The model under review builds one solid part; all positions refer to its coordinate system, in mm. A direction names the side the tool comes from. Coordinates: 2 decimals unless noted, no trailing zeros. Write each loop counter-clockwise with the first axis right and the second up, starting at its lowest first coordinate (ties: lowest second). Pieces come first, ordered by that corner, then holes. Notation, with made-up numbers: (55, 86) - (85, 86) arc R21 cw to (85, 94) - close; hole circle Ø2 at (79.5, 58.25). An arc over 180 degrees is marked (long way). Return JSON: item names as keys, results as strings. Group by question number.
(1) To check wall thickness, follow L1, parallel to Y at x = 0, z = 6.35; L2, parallel to X at y = 55, z = 25.5; L3, parallel to Z at x = 2, y = 54. State the ranges of each line that lie inside material, in increasing order. Write a range as from..to.
(2) We need section D-D on x = 13. State the section outline as (y, z) points, then the cut area to 3 significant figures.
(3) Tool access review of faces 5 (the face through (-29, 33.924, 4)), 6 (the face through (0, 43, 4.25)), 7 (the face through (10.25, 34, 31)): name each direction out of +Z, -Z, +X, -X, +Y, -Y from which nothing blocks a thin tool from reaching the whole face with its end or side.
(4) Draft analysis for pull direction Y (two halves, no side actions). For faces 1 (the face through (-27.766, 32.006, 32.728)), 2 (the face through (-10.25, 34, 4)), 3 (the face through (1.344, 38.032, 29.197)), 4 (the face through (29, 33.924, 4)), state which applies: released by +Y, released by -Y, zero draft, split by the parting line, or undercut.
(5) We need section B-B on z = 17.5. Give the number of separate pieces and of enclosed holes in the cut face, then the cut area to 3 significant figures.
(6) For pin 1 Ø12 at (x, z) = (-35, 22.5) entering from +Y; pin 2 Ø8 at (x, y) = (28.5, 37.5) entering from +Z; pin 3 Ø3 at (x, z) = (30, 26.5) entering from -Y; pin 4 Ø1.5 at (y, z) = (-0.08, 28.5) entering from +X, all flat-tipped, find the tip position at first contact; note any pin that passes through.
(7) We need section A-A on x = 0. State the section outline as (y, z) points (3 decimals), then the cut area to 3 significant figures.
(8) We need section C-C on y = 20. State the section outline as (x, z) points.
```python
from build123d import *

# Parameters (mm, degrees)
EXTRUDE_1_DEPTH       = 35
SKETCH_6_R            = 6
CUT_EXTRUDE_2_DEPTH   = 103.2
SKETCH_7_R            = 5.75
EXTRUDE_3_DEPTH       = 103.2
CUT_EXTRUDE_3_REACH   = 88.478
F_2_5MM_2_D           = 2.5
F_2_5MM_2_CSINK_D     = 2.55
F_2_5MM_2_CSINK_ANGLE = 90
SKETCH_16_W           = 20.2
SKETCH_16_H           = 20.2
CUT_EXTRUDE_5_DEPTH   = 30
SKETCH_15_W           = 20.5
SKETCH_15_H           = 35
CUT_EXTRUDE_6_DEPTH   = 4.25
SKETCH_17_W           = 20.5
SKETCH_17_H           = 35
CUT_EXTRUDE_7_DEPTH   = 4.25
F_5_0MM_1_D           = 5
F_5_0MM_1_CSINK_D     = 5.05
F_5_0MM_1_CSINK_ANGLE = 90
CUT_EXTRUDE_8_REACH   = 126.363
CUT_EXTRUDE_9_DEPTH   = 36.25
CUT_EXTRUDE_10_DEPTH  = 36.25
CUT_EXTRUDE_11_REACH  = 98.427
CUT_EXTRUDE_12_DEPTH  = 87.477815158


with BuildPart() as part:
    # 草图1 → 凸台-拉伸1 (new body)
    with BuildSketch(Plane.XY):
        Polygon((51.6, -0.076277531), (51.6, 29.923722469), (20, 59.923722469), (-20, 59.923722469), (-51.6, 29.923722469), (-51.6, -0.076277531), align=None)
    extrude(amount=EXTRUDE_1_DEPTH)

    # 草图6 → 切除-拉伸2 (cut)
    with BuildSketch(Plane.ZY.offset(51.6)):
        with Locations((17.5, -0.076277531)):
            Circle(SKETCH_6_R)
    extrude(amount=-CUT_EXTRUDE_2_DEPTH, mode=Mode.SUBTRACT)

    # 草图7 → 凸台-拉伸3 (add)
    with BuildSketch(Plane.ZY.offset(51.6)):
        with Locations((5.75, -0.076277531)):
            Circle(SKETCH_7_R)
        with Locations((29.25, -0.076277531)):
            Circle(SKETCH_7_R)
    extrude(amount=-EXTRUDE_3_DEPTH)

    # 切除-拉伸3: up to this face of the body (flat: up to its plane)
    cut_extrude_3_end = Plane(part.part.faces().sort_by_distance((0, 26.308161829, 0))[0])
    # 草图8 → 切除-拉伸3 (cut, up to the picked face)
    with BuildSketch(Plane.XY.offset(35), mode=Mode.PRIVATE) as cut_extrude_3_sk1:
        Polygon((-46.6, -0.076277531), (-46.6, 24.923722469), (46.6, 24.923722469), (46.6, -0.076277531), (46.6, -12.111349377), (-46.6, -12.111349377), align=None)
    cut_extrude_3_tool1 = split(extrude(cut_extrude_3_sk1.sketch, amount=-CUT_EXTRUDE_3_REACH, mode=Mode.PRIVATE), bisect_by=cut_extrude_3_end, keep=Keep.BOTH, mode=Mode.PRIVATE)
    add(cut_extrude_3_tool1.solids().sort_by(Axis((0, 6.406187, 35), (0, 0, -1)))[0], mode=Mode.SUBTRACT)

    # Ø2.5mm 暗销孔2 (through all)
    with Locations(Plane(origin=(51.6, 0, 0), x_dir=(0, 0, -1), z_dir=(1, 0, 0))):
        with Locations((-28.5, -0.076277531), (-25.278174593, 7.701897062), (-17.5, 10.923722469), (-9.721825407, 7.701897062), (-6.5, -0.076277531)):
            CounterSinkHole(F_2_5MM_2_D / 2, F_2_5MM_2_CSINK_D / 2, counter_sink_angle=F_2_5MM_2_CSINK_ANGLE)

    # 草图16 → 切除-拉伸5 (cut)
    with BuildSketch(Plane(origin=(0, 59.923722469, 0), x_dir=(1, 0, 0), z_dir=(0, 1, 0))):
        with Locations((0, -17.5)):
            Rectangle(SKETCH_16_W, SKETCH_16_H)
    extrude(amount=-CUT_EXTRUDE_5_DEPTH, mode=Mode.SUBTRACT)

    # 草图15 → 切除-拉伸6 (cut)
    with BuildSketch(Plane.XY.offset(35)):
        with Locations((0, 42.423722469)):
            Rectangle(SKETCH_15_W, SKETCH_15_H)
    extrude(amount=-CUT_EXTRUDE_6_DEPTH, mode=Mode.SUBTRACT)

    # 草图17 → 切除-拉伸7 (cut)
    with BuildSketch(Plane(origin=(0, 0, 0), x_dir=(-1, 0, 0), z_dir=(0, 0, -1))):
        with Locations((0, 42.423722469)):
            Rectangle(SKETCH_17_W, SKETCH_17_H)
    extrude(amount=-CUT_EXTRUDE_7_DEPTH, mode=Mode.SUBTRACT)

    # Ø5.0mm 暗销孔1 (through all)
    with Locations(Plane(origin=(0, 0, 4.25), x_dir=(-1, 0, 0), z_dir=(0, 0, -1))):
        with Locations((0, 50.923722469), (0, 35.923722469)):
            CounterSinkHole(F_5_0MM_1_D / 2, F_5_0MM_1_CSINK_D / 2, counter_sink_angle=F_5_0MM_1_CSINK_ANGLE)

    # 切除-拉伸8: up to this face of the body (flat: up to its plane)
    cut_extrude_8_end = Plane(part.part.faces().sort_by_distance((-51.6, 14.113222329, 17.5))[0])
    # 草图20 → 切除-拉伸8 (cut, up to the picked face)
    with BuildSketch(Plane(origin=(51.6, 0, 0), x_dir=(0, 0, -1), z_dir=(1, 0, 0)), mode=Mode.PRIVATE) as cut_extrude_8_sk1:
        Polygon((-30.75, 59.923722469), (-35, 59.923722469), (-35, -0.076277531), align=None)
    cut_extrude_8_tool1 = split(extrude(cut_extrude_8_sk1.sketch, amount=-CUT_EXTRUDE_8_REACH, mode=Mode.PRIVATE), bisect_by=cut_extrude_8_end, keep=Keep.BOTH, mode=Mode.PRIVATE)
    # 草图20 → 切除-拉伸8 (cut, up to the picked face)
    with BuildSketch(Plane(origin=(51.6, 0, 0), x_dir=(0, 0, -1), z_dir=(1, 0, 0)), mode=Mode.PRIVATE) as cut_extrude_8_sk2:
        Polygon((0, -0.076277531), (0, 59.923722469), (-4.25, 59.923722469), align=None)
    cut_extrude_8_tool2 = split(extrude(cut_extrude_8_sk2.sketch, amount=-CUT_EXTRUDE_8_REACH, mode=Mode.PRIVATE), bisect_by=cut_extrude_8_end, keep=Keep.BOTH, mode=Mode.PRIVATE)
    add(cut_extrude_8_tool1.solids().sort_by(Axis((51.6, 39.923722, 33.583333), (-1, 0, 0)))[0], mode=Mode.SUBTRACT)
    add(cut_extrude_8_tool2.solids().sort_by(Axis((51.6, 39.923722, 1.416667), (-1, 0, 0)))[0], mode=Mode.SUBTRACT)

    # 草图21 → 切除-拉伸9 (cut)
    with BuildSketch(Plane(origin=(51.6, 0, 0), x_dir=(0, 0, -1), z_dir=(1, 0, 0))):
        Polygon((-27.6, 59.923722469), (-29.725, 29.923722469), (-5.275, 29.923722469), (-7.4, 59.923722469), align=None)
    extrude(amount=-CUT_EXTRUDE_9_DEPTH, mode=Mode.SUBTRACT)

    # 草图22 → 切除-拉伸10 (cut)
    with BuildSketch(Plane.ZY.offset(51.6)):
        Polygon((29.725, 29.923722469), (27.6, 59.923722469), (7.4, 59.923722469), (5.275, 29.923722469), align=None)
    extrude(amount=-CUT_EXTRUDE_10_DEPTH, mode=Mode.SUBTRACT)

    # 切除-拉伸11: up to this face of the body (flat: up to its plane)
    cut_extrude_11_end = Plane(part.part.faces().sort_by_distance((15.35, 44.447798617, 17.5))[0])
    # 草图23 → 切除-拉伸11 (cut, up to the picked face)
    with BuildSketch(Plane.ZY.offset(15.35), mode=Mode.PRIVATE) as cut_extrude_11_sk1:
        with BuildLine():
            Line((13.5, 34.923722469), (21.5, 34.923722469))
            ThreePointArc((21.5, 34.923722469), (23.621320344, 35.802402126), (24.5, 37.923722469))
            Line((24.5, 37.923722469), (24.5, 51.923722469))
            ThreePointArc((24.5, 51.923722469), (23.621320344, 54.045042813), (21.5, 54.923722469))
            Line((21.5, 54.923722469), (13.5, 54.923722469))
            ThreePointArc((13.5, 54.923722469), (11.378679656, 54.045042813), (10.5, 51.923722469))
            Line((10.5, 51.923722469), (10.5, 37.923722469))
            ThreePointArc((10.5, 37.923722469), (11.378679656, 35.802402126), (13.5, 34.923722469))
        make_face()
    cut_extrude_11_tool1 = split(extrude(cut_extrude_11_sk1.sketch, amount=-CUT_EXTRUDE_11_REACH, mode=Mode.PRIVATE), bisect_by=cut_extrude_11_end, keep=Keep.BOTH, mode=Mode.PRIVATE)
    add(cut_extrude_11_tool1.solids().sort_by(Axis((-15.35, 44.923722, 17.5), (1, 0, 0)))[0], mode=Mode.SUBTRACT)

    # 草图25 → 切除-拉伸12 (cut, through all)
    with BuildSketch(Plane.XY):
        Polygon((39.35, 33.923722469), (19.35, 33.923722469), (19.35, 52.911064241), align=None)
        Polygon((-19.35, 52.911064241), (-39.35, 33.923722469), (-19.35, 33.923722469), align=None)
    extrude(amount=CUT_EXTRUDE_12_DEPTH, mode=Mode.SUBTRACT)


solid = part.part
```
Ans:
{
 "1": {"L1": "24.92..33.42, 38.42..48.42, 53.42..59.92", "L2": "-15.35..-10.1, 10.1..15.35", "L3": "4.25..7.4, 27.6..30.75"},
 "2": {"outline": "(24.92, 1.77) - (59.92, 4.25) - (59.92, 30.75) - (24.92, 33.23) - close; hole (34.92, 13.5) arc R3 ccw to (37.92, 10.5) - (51.92, 10.5) arc R3 ccw to (54.92, 13.5) - (54.92, 21.5) arc R3 ccw to (51.92, 24.5) - (37.92, 24.5) arc R3 ccw to (34.92, 21.5) - close", "area": "742 mm²"},
 "3": {"face 5": "+Z, -Z", "face 6": "-Z, +Y, -Y", "face 7": "+Z, +Y, -Y"},
 "4": {"face 1": "released by +Y", "face 2": "zero draft", "face 3": "undercut", "face 4": "undercut"},
 "5": {"separate pieces": "5", "enclosed holes": "0", "area": "786 mm²"},
 "6": {"pin 1": "y = 29.92", "pin 2": "z = 32.62", "pin 3": "y = 24.92", "pin 4": "through"},
 "7": {"outline": "(24.924, 4.25) - (33.399, 4.25) - (33.424, 4.275) - (33.424, 7.4) - (29.924, 7.4) - (29.924, 27.6) - (33.424, 27.6) - (33.424, 30.75) - (24.924, 30.75) - close; (38.424, 4.275) - (38.449, 4.25) - (48.399, 4.25) - (48.424, 4.275) - (48.424, 7.4) - (38.424, 7.4) - close; (38.424, 27.6) - (48.424, 27.6) - (48.424, 30.75) - (38.424, 30.75) - close; (53.424, 4.275) - (53.449, 4.25) - (59.924, 4.25) - (59.924, 7.4) - (53.424, 7.4) - close; (53.424, 27.6) - (59.924, 27.6) - (59.924, 30.75) - (53.424, 30.75) - close", "area": "258 mm²"},
 "8": {"outline": "(-51.6, 1.42) - (-46.6, 1.42) - (-46.6, 33.58) - (-51.6, 33.58) - close; (46.6, 1.42) - (51.6, 1.42) - (51.6, 33.58) - (46.6, 33.58) - close"}
}
